```python
from build123d import *

# Parameters (mm, degrees)
SKETCH1_W             = 6
SKETCH1_H             = 80
ROD_BAR_DEPTH         = 2
LINK_HOLES_DEPTH      = 41.162171256
LINK_HOLES_DEPTH_BACK = 41.162171256
SKETCH2_R             = 1.3
SKETCH3_R             = 0.8
SMA_SPRING_PEG_DEPTH  = 3
BIAS_SPRING_PEG_START = 3
SKETCH4_R             = 0.8
BIAS_SPRING_PEG_DEPTH = 3


with BuildPart() as part:
    # Sketch1 → Rod_Bar (new body)
    with BuildSketch(Plane.XY):
        Rectangle(SKETCH1_W, SKETCH1_H)
    extrude(amount=ROD_BAR_DEPTH)

    # Sketch2 → Link_Holes (cut, two sides: drawn at the far end of the back side and taken through both)
    with BuildSketch(Plane.XY.offset(-LINK_HOLES_DEPTH_BACK)):
        with Locations((0, -30)):
            Circle(SKETCH2_R)
        with Locations((0, -10)):
            Circle(SKETCH2_R)
        with Locations((0, 10)):
            Circle(SKETCH2_R)
        with Locations((0, 30)):
            Circle(SKETCH2_R)
    extrude(amount=LINK_HOLES_DEPTH + LINK_HOLES_DEPTH_BACK, mode=Mode.SUBTRACT)

    # Sketch3 → SMA_Spring_Peg (add)
    with BuildSketch(Plane(origin=(0, 40, 0), x_dir=(1, 0, 0), z_dir=(0, 1, 0))):
        with Locations(Location((0, -1, 0), (0, 0, 270))):
            Circle(SKETCH3_R)
    extrude(amount=SMA_SPRING_PEG_DEPTH)

    # Sketch4 → Bias_Spring_Peg (add)
    with BuildSketch(Plane.XZ.offset(40).offset(BIAS_SPRING_PEG_START)):
        with Locations(Location((0, 1, 0), (0, 0, 90))):
            Circle(SKETCH4_R)
    extrude(amount=-BIAS_SPRING_PEG_DEPTH)


solid = part.part
```
Could you check a few things on this model? Use its own coordinates, in mm. A direction names the side the tool comes from. Round coordinates to 2 decimals unless told otherwise and drop trailing zeros. Loops run counter-clockwise (first coordinate to the right, second up) from the corner with the lowest first, then second, coordinate; pieces in that order, holes last. Notation, with made-up numbers: M -40,30 L -10,30 A24 ccw -10,45 Z; hole C 77,50.25 d1. An arc over 180 degrees is marked long. Put each result on its own line as item: value.
Q1. Thinking about a two-plate mould opening in X: for faces 1 (the face through (-0.17, -8.71, 0.99)), 2 (the face through (-3, -1, 1)), 3 (the face through (0, 1, 0)), which applies, released by +X, released by -X, zero draft, split by the parting line, or undercut?
Check result:
face 1: undercut
face 2: released by -X
face 3: zero draft
Q2. For pin 1 (1 mm diameter, centred on x = -1.5, z = 1.5, fed in from +Y); pin 2 (3.5 mm diameter, centred on x = 0, y = -30, fed in from -Z), each with a flat end and sliding along its axis, tell me the tip position at first contact or that it passes through.
Check result:
pin 1: y = 40
pin 2: z = 0
Q3. Imagine slicing it at C-C (y = -10). Write out the boundary of the cut face in (x, z).
Check result:
outline: M -3,0 L -1.3,0 L -1.3,2 L -3,2 Z; M 1.3,0 L 3,0 L 3,2 L 1.3,2 Z
Q4. On a 3-axis mill with a long thin cutter (end or side, diameter ignored), from which of +Z, -Z, +X, -X, +Y, -Y can I reach the whole of each face in a straight line? I mean faces 4 (the face through (0, 1, 2)), 5 (the face through (-0.49, 41.48, 0.37)), 6 (the face through (0.49, -41.52, 0.37)). Say none if no direction works.
Check result:
face 4: +Z, +X, -X, +Y, -Y
face 5: +Y
face 6: -Y
Q5. Imagine slicing it at A-A (x = 0). Write out the boundary of the cut face in (y, z).
Check result:
outline: M -43,0.2 L -40,0.2 L -40,0 L -31.3,0 L -31.3,2 L -40,2 L -40,1.8 L -43,1.8 Z; M -28.7,0 L -11.3,0 L -11.3,2 L -28.7,2 Z; M -8.7,0 L 8.7,0 L 8.7,2 L -8.7,2 Z; M 11.3,0 L 28.7,0 L 28.7,2 L 11.3,2 Z; M 31.3,0 L 40,0 L 40,0.2 L 43,0.2 L 43,1.8 L 40,1.8 L 40,2 L 31.3,2 Z
Q6. I need wall thicknesses on probe 1 along Y at (x, z) = (0, 0.55); probe 2 along X at (y, z) = (10, 1.15); probe 3 along Y at (x, z) = (-0.5, 0.6). Which ranges of each line are inside material? Lowest first, please.
Check result:
probe 1: -43 to -31.3, -28.7 to -11.3, -8.7 to 8.7, 11.3 to 28.7, 31.3 to 43
probe 2: -3 to -1.3, 1.3 to 3
probe 3: -43 to -31.2, -28.8 to -11.2, -8.8 to 8.8, 11.2 to 28.8, 31.2 to 43
Q7. Imagine slicing it at B-B (z = 1). Write out the boundary of the cut face in (x, y), then the cut area to 3 significant figures.
Check result:
outline: M -3,-40 L -0.8,-40 L -0.8,-43 L 0.8,-43 L 0.8,-40 L 3,-40 L 3,40 L 0.8,40 L 0.8,43 L -0.8,43 L -0.8,40 L -3,40 Z; hole C 0,-30 d2.6; hole C 0,-10 d2.6; hole C 0,10 d2.6; hole C 0,30 d2.6
area: 468 mm2
